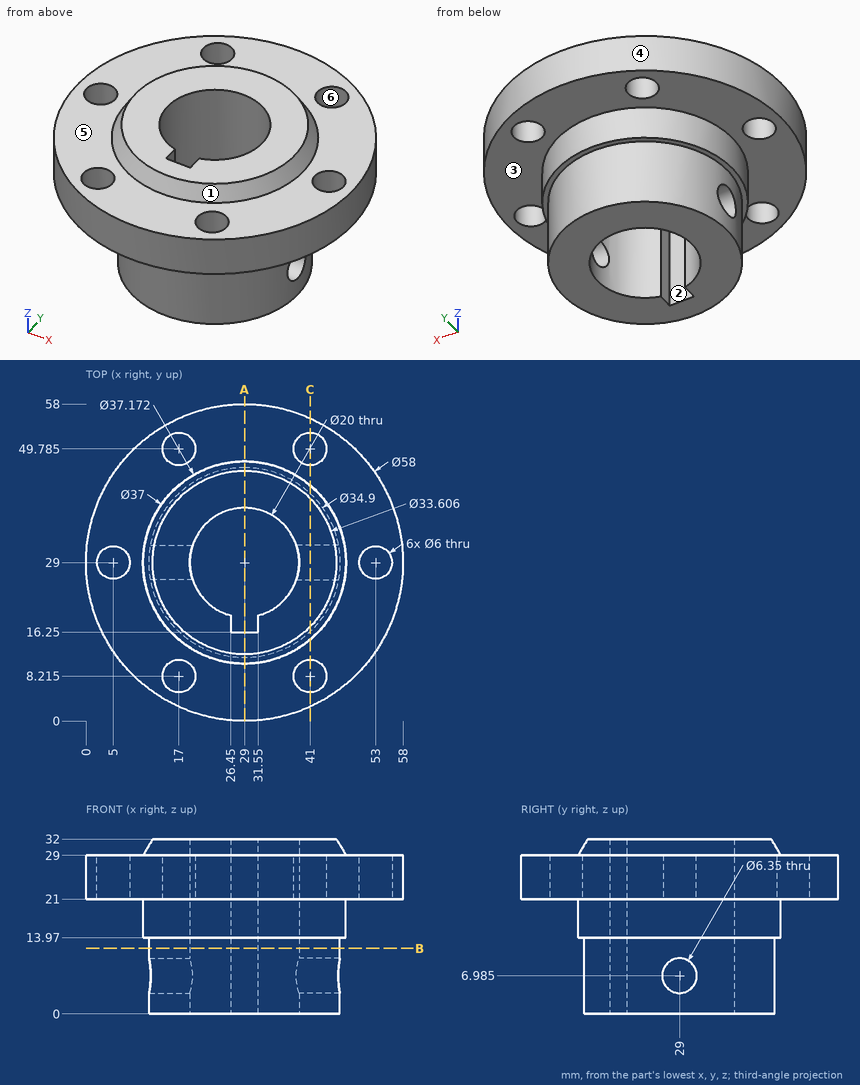
Check sheet for the drawn part. Datum: minimum x, y, z corner. Units: mm. A direction names the side the tool comes from. Give positions to 0.01 mm unless a question says otherwise; leave off trailing zeros. Order: outer loops, then holes, each group sorted by start corner. A loop starts at its lowest first (then second) coordinate and runs counter-clockwise, first axis right, second up. Notation, with made-up numbers: (21, -28) - (61, -28) arc R28 cw to (61, 5) - close; hole circle Ø4 at (7, 45.25). An arc over 180 degrees is marked (long way). Write item = value, one per line. Start each with the question number.
1) Access from +Z, -Z, +X, -X, +Y, -Y to the whole of each face (thin tool, end or side, straight path). Record for the marked faces 1, 2 and 3.
2) Gauge pin test, flat ends, axial feed: pin 1 Ø6 at (y, z) = (40, 20) entering from +X (1 decimal); pin 2 Ø10 at (x, z) = (21, 26) entering from +Y (1 decimal); pin 3 Ø16 at (x, y) = (29, 29) entering from +Z; pin 4 Ø12 at (y, z) = (20, 15.5) entering from -X. Record the tip position at first contact, or that the pin passes through.
3) Section check A-A (x = 29). Enter the section's corners in (y, z).
4) Scan lines: L1, parallel to Y at x = 41, z = 24 (1 decimal); L2, parallel to Z at x = 13, y = 39; L3, parallel to Z at x = 43, y = 29. Record each from-to range of solid material in increasing order.
5) Section check B-B (z = 12). Enter the section's corners in (x, y), then the cut area to 3 significant figures.
6) Section check C-C (x = 41). Count the separate pieces of the cut face and the enclosed holes in it.
7) Draft check along Y on the marked faces 4, 5 and 6. Enter one of: released by +Y, released by -Y, zero draft, split by the parting line, or undercut.
Geometry check:
q1.face_1 = +Z
q1.face_2 = +Z, -Z
q1.face_3 = -Z
q2.pin_1 = 56.8
q2.pin_2 = 57.8
q2.pin_3 = through
q2.pin_4 = 0.76
q3.outline = (0, 21) - (10.5, 21) - (10.5, 13.97) - (11.55, 13.97) - (11.55, 0) - (16.25, 0) - (16.25, 32) - (12.2, 32) - (10.41, 29) - (0, 29) - close; (39, 0) - (46.45, 0) - (46.45, 13.97) - (47.5, 13.97) - (47.5, 21) - (58, 21) - (58, 29) - (47.59, 29) - (45.8, 32) - (39, 32) - close
q4.L1 = 2.6 to 5.2, 11.2 to 46.8, 52.8 to 55.4
q4.L2 = 21 to 29
q4.L3 = 0 to 3.81, 10.16 to 32
q5.outline = circle Ø34.9 at (29, 29); hole (26.45, 16.25) - (31.55, 16.25) - (31.55, 19.33) arc R10 ccw (long way) to (26.45, 19.33) - close
q5.area = 628 mm2
q6.separate_pieces = 3
q6.enclosed_holes = 1
q7.face_4 = split by the parting line
q7.face_5 = zero draft
q7.face_6 = undercut
